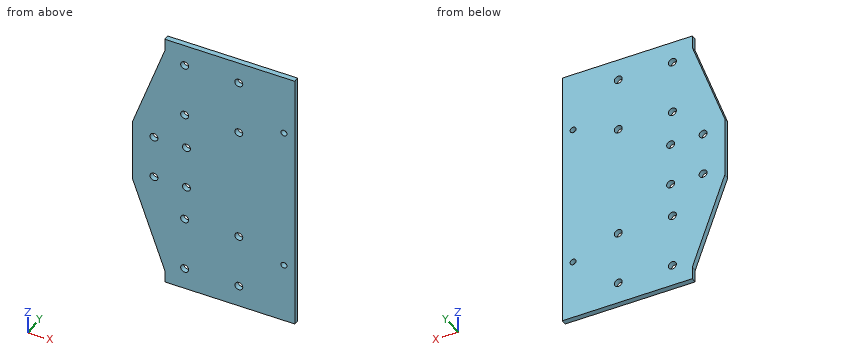
from build123d import *

# Parameters (mm, degrees)
EXTRUDE_1_DEPTH     = 3
SKETCH_2_R          = 2.2
SKETCH_2_R_2        = 1.65
CUT_EXTRUDE_1_DEPTH = 10


with BuildPart() as part:
    # 草图1 → 凸台-拉伸1 (new body)
    with BuildSketch(Plane(origin=(0, 0, 0), x_dir=(1, 0, 0), z_dir=(0, 1, 0))):
        Polygon((0, 0), (29.84652885, 0), (29.84652885, 147), (0, 147), (-42.15347115, 147), (-42.15347115, 140), (-60.15347115, 90.5), (-60.15347115, 56.5), (-42.15347115, 7), (-42.15347115, 0), align=None)
    extrude(amount=EXTRUDE_1_DEPTH)

    # 草图2 → 切除-拉伸1 (cut)
    with BuildSketch(Plane(origin=(0, 3, 0), x_dir=(1, 0, 0), z_dir=(0, 1, 0))):
        with Locations(Location((-48.15347115, 85.5, 0), (0, 0, 270))):
            Circle(SKETCH_2_R)
        with Locations(Location((-30.15347115, 85.5, 0), (0, 0, 270))):
            Circle(SKETCH_2_R)
        with Locations(Location((-30.15347115, 61.5, 0), (0, 0, 270))):
            Circle(SKETCH_2_R)
        with Locations(Location((-48.15347115, 61.5, 0), (0, 0, 270))):
            Circle(SKETCH_2_R)
        with Locations(Location((-1.15347115, 135, 0), (0, 0, 270))):
            Circle(SKETCH_2_R)
        with Locations(Location((-1.15347115, 105, 0), (0, 0, 270))):
            Circle(SKETCH_2_R)
        with Locations(Location((-31.15347115, 135, 0), (0, 0, 270))):
            Circle(SKETCH_2_R)
        with Locations(Location((-31.15347115, 105, 0), (0, 0, 270))):
            Circle(SKETCH_2_R)
        with Locations(Location((-31.15347115, 42, 0), (0, 0, 270))):
            Circle(SKETCH_2_R)
        with Locations(Location((-31.15347115, 12, 0), (0, 0, 270))):
            Circle(SKETCH_2_R)
        with Locations(Location((-1.15347115, 42, 0), (0, 0, 270))):
            Circle(SKETCH_2_R)
        with Locations(Location((-1.15347115, 12, 0), (0, 0, 270))):
            Circle(SKETCH_2_R)
        with Locations(Location((23.84652885, 113.5, 0), (0, 0, 270))):
            Circle(SKETCH_2_R_2)
        with Locations(Location((23.84652885, 33.5, 0), (0, 0, 270))):
            Circle(SKETCH_2_R_2)
    extrude(amount=-CUT_EXTRUDE_1_DEPTH, mode=Mode.SUBTRACT)


solid = part.part
Source: CAD feature listing. Evaluate the final solid. Frame: model axes, mm. Round coordinates to 2 decimals unless told otherwise and drop trailing zeros. Loops run counter-clockwise (first coordinate to the right, second up) from the corner with the lowest first, then second, coordinate; pieces in that order, holes last. Notation, with made-up numbers: (84, -15) - (99, -15) arc R21 ccw to (99, -5) - close; hole circle Ø3 at (59.25, 16). An arc over 180 degrees is marked (long way). Write item = value, one per line. Start each with the question number.
(1) Ray query, line 1 along Z through (x, y) = (-1, 1); line 2 along X through (y, z) = (2.7, -87.5); line 3 along X through (y, z) = (1.2, -135). Return the intervals inside material, ascending. Write a range as from..to.
(2) Section query D-D, the plane z = -126. Output: boundary loops of the cut face in (x, y).
(3) Section query C-C, the plane z = -12. Output: boundary loops of the cut face in (x, y).
(4) Pin query (flat end, axial travel): pin 1 (4.5 mm diameter, centred on x = 23.85, z = -113.5, fed in from +Y). Return the tip coordinate at first contact, or that it passes through.
(5) Section query A-A, the plane z = -33.5. Output: boundary loops of the cut face in (x, y).
(6) Section query B-B, the plane y = 0.7. State how many separate pieces and enclosed holes the cut face has, plus the area to 3 significant figures.
Conclusion:
q1.line_1 = -147..-137.19, -132.81..-107.19, -102.81..-44.19, -39.81..-14.19, -9.81..0
q1.line_2 = -60.15..-49.07, -47.24..-31.07, -29.24..29.85
q1.line_3 = -43.97..-33.35, -28.95..-3.35, 1.05..29.85
q2.outline = (-47.24, 0) - (29.85, 0) - (29.85, 3) - (-47.24, 3) - close
q3.outline = (-43.97, 0) - (-33.35, 0) - (-33.35, 3) - (-43.97, 3) - close; (-28.95, 0) - (-3.35, 0) - (-3.35, 3) - (-28.95, 3) - close; (1.05, 0) - (29.85, 0) - (29.85, 3) - (1.05, 3) - close
q4.pin_1 = 3
q5.outline = (-51.79, 0) - (22.2, 0) - (22.2, 3) - (-51.79, 3) - close; (25.5, 0) - (29.85, 0) - (29.85, 3) - (25.5, 3) - close
q6.separate_pieces = 1
q6.enclosed_holes = 14
q6.area = 11,900 mm2
